Verification items for the finished model (mm, model axes). A direction names the side the tool comes from. Coordinates: 2 decimals unless noted, no trailing zeros. Write each loop counter-clockwise with the first axis right and the second up, starting at its lowest first coordinate (ties: lowest second). Pieces come first, ordered by that corner, then holes. Notation, with made-up numbers: M 58,-26.75 L 96,-26.75 A18 cw 96,-12.75 Z; hole C -22.5,74.25 d8. An arc over 180 degrees is marked long. Answer in a Markdown table with one row per item.
Autodesk Inventor part; units mm, degrees
ref_plane "Work Plane1" through (0, 0, 5) normal (0, 0, 1) x (1, 0, 0)
ref_plane "YZ Plane" through (0, 0, 0) normal (1, 0, 0) x (0, 1, 0)
ref_plane "XZ Plane" through (0, 0, 0) normal (0, 1, 0) x (-1, 0, 0)
sketch "Sketch2" plane through (0, 0, 0) normal (0, 0, 1) x (1, 0, 0)
  circle A0 centre (0, 0) radius 6
  dimension "d0" = 12
ref_plane "Work Plane1" through (0, 0, 5) normal (0, 0, 1) x (1, 0, 0)
sketch "Sketch3" plane through (0, 0, 5) normal (0, 0, 1) x (1, 0, 0)
  circle A0 centre (0, 0) radius 4.5
  dimension "d2" = 9
loft "Loft1" add profiles "Sketch2", "Sketch3"
sketch "Sketch4" plane through (0, 0, 0) normal (0, 0, -1) x (-1, 0, 0)
  circle A0 centre (0, 0) radius 6
extrude "Extrusion1" add sketch "Sketch4" along normal blind 1
sketch "Sketch5" plane through (0, 0, -1) normal (0, 0, -1) x (-1, 0, 0)
  circle A0 centre (0, 0) radius 4
  dimension "d9" = 8
extrude "Extrusion2" add sketch "Sketch5" along normal blind 12
sketch "Sketch6" plane through (0, 0, -13) normal (0, 0, -1) x (-1, 0, 0)
  circle A0 centre (0, 0) radius 3.1
  dimension "d12" = 6.2
extrude "Extrusion3" add sketch "Sketch6" along normal blind 4
properties part number "driver gear"
1) Thickness scan on L1, parallel to Z at x = 1, y = 4; L2, parallel to Z at x = -3.75, y = 1; L3, parallel to X at y = 0.25, z = -4.75. Record the ranges inside material, lowest first. Write a range as [from, to].
Response values:
| item | result |
|---|---|
| L1 | z = [-1, 5] |
| L2 | z = [-13, 5] |
| L3 | x = [-3.99, 3.99] |
2) Sectioned sample at B-B (z = 3). Record the cut outline in (x, y), then the cut area to 3 significant figures.
Response values:
| item | result |
|---|---|
| outline | C 0,0 d10.2 |
| area | 81.7 mm² |
3) Sectioned sample at A-A (x = 0). Record the cut outline in (y, z).
Response values:
| item | result |
|---|---|
| outline | M -6,-1 L -4,-1 L -4,-13 L -3.1,-13 L -3.1,-17 L 3.1,-17 L 3.1,-13 L 4,-13 L 4,-1 L 6,-1 L 6,0 L 4.5,5 L -4.5,5 L -6,0 Z |
4) Sectioned sample at C-C (z = -14). Record the cut outline in (x, y).
Response values:
| item | result |
|---|---|
| outline | C 0,0 d6.2 |
5) Depth check by flat-ended pin: pin 1 (3 mm diameter, centred on y = -3, z = -7, fed in from -X); pin 2 (6 mm diameter, centred on x = -2.5, y = -4.5, fed in from -Z); pin 3 (2 mm diameter, centred on x = 2.5, z = -4, fed in from -Y). Enter the tip coordinate at first touch or a pass-through.
Response values:
| item | result |
|---|---|
| pin 1 | stops at x = -3.71 |
| pin 2 | stops at z = -17 |
| pin 3 | stops at y = -3.71 |
6) Tool access check on faces 1 (the face through (0, 0, 5)), 2 (the face through (-1.43, 2.75, -14.97)). Record the directions out of +Z, -Z, +X, -X, +Y, -Y that give a thin tool (end or side, any length) a straight path to the whole face; none if there is none.
Response values:
| item | result |
|---|---|
| face 1 | +Z, +X, -X, +Y, -Y |
| face 2 | -Z |
